from build123d import *

# Parameters (mm, degrees)
SKETCH_2_R          = 40
CUT_EXTRUDE_1_DEPTH = 4


with BuildPart() as part:
    # 草图1 → 旋转1 (revolve)
    with BuildSketch(Plane.XY, mode=Mode.PRIVATE) as revolve_1_sk:
        Polygon((0, 9.5), (0, 7.5), (0.812, 6.688), (3.188, 6.688), (4, 7.5), (4, 9.5), (2.472689603, 15.2), (1.527310397, 15.2), align=None)
    revolve(revolve_1_sk.sketch.rotate(Axis((4, 0, 0), (-1, 0, 0)), 270), axis=Axis((4, 0, 0), (-1, 0, 0)))

    # 草图2 → 切除-拉伸1 (cut)
    with BuildSketch(Plane(origin=(0, 0, 0), x_dir=(0, 0, -1), z_dir=(1, 0, 0))):
        Circle(SKETCH_2_R)
        Polygon((-9.5, -5.484827557), (0, -10.969655115), (9.5, -5.484827557), (9.5, 5.484827557), (0, 10.969655115), (-9.5, 5.484827557), align=None, mode=Mode.SUBTRACT)
    extrude(amount=CUT_EXTRUDE_1_DEPTH, mode=Mode.SUBTRACT)


solid = part.part
Part model, mm, in its own coordinate system. Coordinates: 2 decimals unless noted, no trailing zeros. Order: outer loops, then holes, each group sorted by start corner. A loop starts at its lowest first (then second) coordinate and runs counter-clockwise, first axis right, second up. Notation, with made-up numbers: (18.5, -5.75) - (63.5, -5.75) arc R27 ccw to (63.5, 31.25) - close; hole circle Ø7 at (-21.5, -37). An arc over 180 degrees is marked (long way). Use CSV: the item, a comma, the result in double quotes.
Item 1: Mould opens along Z. For faces 1 (the face through (1.972, 8.266, 4.684)), 2 (the face through (2.02, 2.01, 6.38)), 3 (the face through (1.972, -8.266, -4.684)), 4 (the face through (0.094, 9.85, 0.024)) say: +Z half, -Z half, draft (parallel to the pull), parting line (faces both ways), or undercut.
Solved:
face 1,"+Z half"
face 2,"undercut"
face 3,"-Z half"
face 4,"parting line"
Item 2: Drop flat-ended pins along their axis: P1, Ø5, axis at y = -1, z = 7, coming from the -X side; P2, Ø1.5, axis at y = -4.5, z = 4.5, coming from the -X side; P3, Ø8, axis at y = 0, z = 0, coming from the -X side. Give the stop position or say it passes through.
Solved:
P1,"stops at x = 0"
P2,"stops at x = 0.39"
P3,"passes through"
Item 3: Saw through at A-A on x = 2.1. Give the cut face in (y, z), and give its area (3 significant figures).
Solved:
outline,"(-10.97, 0) - (-5.48, -9.5) - (5.48, -9.5) - (10.97, 0) - (5.48, 9.5) - (-5.48, 9.5) - close; hole circle Ø13.38 at (0, 0)"
area,"172 mm²"
Item 4: Probe probe 1 along Z at (x, y) = (3.45, 4.75); probe 2 along Y at (x, z) = (2.25, -0.25); probe 3 along Z at (x, y) = (0.55, 5.5). List the from-to ranges inside material, lowest first.
Solved:
probe 1,"z = -9.5 to -5.07, 5.07 to 9.5"
probe 2,"y = -10.83 to -6.68, 6.68 to 10.83"
probe 3,"z = -9.47 to -4.25, 4.25 to 9.47"
